from build123d import *

# Parameters (mm, degrees)
F0_W           = 1000
F0_H           = 125
F1_DEPTH       = 25
F2_W           = 820
F2_H           = 17
F3_DEPTH       = 23
F4_R           = 4
F5_DEPTH       = 25
F6_W           = 100
F6_H           = 80
F7_DEPTH       = 35
F8_W           = 50
F8_H           = 10
F9_DEPTH       = 10
F10_W          = 10
F10_H          = 60
F10_R          = 2.5
F11_DEPTH      = 10
F13_DEPTH      = 20
F13_DEPTH_BACK = 30
F14_R          = 5
F15_DEPTH      = 25
F17_W          = 1
F17_H          = 125
F18_DEPTH      = 1


with BuildPart() as f1:
    # F0 (on Top) → F1 (new body)
    with BuildSketch(Plane.XY):
        with Locations((500, 62.5)):
            Rectangle(F0_W, F0_H)
    extrude(amount=F1_DEPTH)

    # F2 (on face) → F3 (join)
    with BuildSketch(Plane.XY.offset(25)):
        with Locations((590, 50)):
            Rectangle(F2_W, F2_H)
    extrude(amount=F3_DEPTH)

    # F4 (on face) → F5 (cut, through all)
    with BuildSketch(Plane.XY.offset(25)):
        with Locations((312, 20)):
            Circle(F4_R)
        with Locations((332, 20)):
            Circle(F4_R)
    extrude(amount=-F5_DEPTH, mode=Mode.SUBTRACT)

    # F6 (on face) → F7 (join)
    with BuildSketch(Plane.XY.offset(25)):
        with Locations((130, 50)):
            Rectangle(F6_W, F6_H)
    extrude(amount=F7_DEPTH)

    # F8 (on face) → F9 (join)
    with BuildSketch(Plane.XY.offset(60)):
        with Locations((82, 50)):
            Rectangle(F8_W, F8_H)
    extrude(amount=F9_DEPTH)

    # F10 (on face) → F11 (join)
    with BuildSketch(Plane(origin=(57, 0, 0), x_dir=(0, -1, 0), z_dir=(-1, 0, 0))):
        with Locations((-60, 65)):
            Rectangle(F10_W, F10_H)
        with Locations((-60, 90)):
            Circle(F10_R, mode=Mode.SUBTRACT)
        with Locations((-40, 65)):
            Rectangle(F10_W, F10_H)
        with Locations((-40, 90)):
            Circle(F10_R, mode=Mode.SUBTRACT)
    extrude(amount=-F11_DEPTH)

    # F12 (on face) → F13 (join, two sides)
    with BuildSketch(Plane.XZ.offset(-45)) as f13_sk:
        Polygon((112, 60), (172, 60), (172, 70), (120, 70), (120, 100), (112, 100), align=None)
    extrude(amount=F13_DEPTH)
    extrude(f13_sk.sketch, amount=-F13_DEPTH_BACK)

    # F14 (on face) → F15 (cut)
    with BuildSketch(Plane.YZ.offset(120)):
        with Locations((40, 90)):
            Circle(F14_R)
        with Locations((60, 90)):
            Circle(F14_R)
    extrude(amount=-F15_DEPTH, mode=Mode.SUBTRACT)

    # F17 (on face) → F18 (join)
    with BuildSketch(Plane.XY.offset(25)):
        with Locations((306.5, 62.5)):
            Rectangle(F17_W, F17_H)
    extrude(amount=F18_DEPTH)


solid = f1.part
Could you check a few things on this model? Use its own coordinates, in mm. A direction names the side the tool comes from. Give positions to 0.01 mm unless a question says otherwise; leave off trailing zeros. Order: outer loops, then holes, each group sorted by start corner. A loop starts at its lowest first (then second) coordinate and runs counter-clockwise, first axis right, second up. Notation, with made-up numbers: (-8.75, 52.25) -> (43.25, 52.25) arc R26 cw to (43.25, 75.25) -> close; hole circle Ø11 at (31, -17). An arc over 180 degrees is marked (long way). Return JSON: item names as keys, results as strings.
1. For pin 1 Ø11 at (x, z) = (63.5, 66) entering from -Y; pin 2 Ø1.1 at (x, y) = (306.5, 104.5) entering from +Z; pin 3 Ø5 at (x, z) = (547.5, 19.5) entering from -Y; pin 4 Ø8 at (x, y) = (253, 61.5) entering from +Z, each with a flat end and sliding along its axis, tell me the tip position at first contact or that it passes through.
Answer list:
{"pin 1": "stops at y = 35", "pin 2": "stops at z = 26", "pin 3": "stops at y = 0", "pin 4": "stops at z = 48"}
2. Thinking about a two-plate mould opening in X: for faces 6 (the flat face through (584, 50, 48)), 7 (the flat face through (1000, 62, 13)), 8 (the flat face through (80, 49, 42)), 9 (the flat face through (57, 50, 65)), which applies, pulls with the +X half, pulls with the -X half, needs draft (parallel to the pull), parting line crosses it, or undercut?
Answer list:
{"face 6": "needs draft", "face 7": "pulls with the +X half", "face 8": "undercut", "face 9": "pulls with the -X half"}
3. I need wall thicknesses on line 1 (Z direction, x = 63.5, y = 60); line 2 (Z direction, x = 114.75, y = 60); line 3 (X direction, y = 37, z = 55.5). Which ranges of each line are inside material? Lowest first, please. Write a range as from..to.
Answer list:
{"line 1": "z = 0..25, 35..87.5, 92.5..95", "line 2": "z = 0..85, 95..100", "line 3": "x = 57..67, 80..180"}
4. On a 3-axis mill with a long thin cutter (end or side, diameter ignored), from which of +Z, -Z, +X, -X, +Y, -Y can I reach the whole of each face in a straight line? I mean faces 1 (the flat face through (135.2, 25, 69.7)), 2 (the flat face through (120, 50, 85)), 3 (the flat face through (135.2, 75, 69.7)), 4 (the flat face through (107, 59, 60)), 5 (the flat face through (112, 50, 80)). Say none if no direction works.
Answer list:
{"face 1": "+Z, +X, -X, -Y", "face 2": "+Z, +X, +Y, -Y", "face 3": "+Z, +X, -X, +Y", "face 4": "+Z", "face 5": "+Z, +Y, -Y"}
5. Imagine slicing it at A-A on x = 866.5. List the corners of the cut face in (y, z) for me.
Answer list:
{"outline": "(0, 0) -> (125, 0) -> (125, 25) -> (58.5, 25) -> (58.5, 48) -> (41.5, 48) -> (41.5, 25) -> (0, 25) -> close"}
